```python
from build123d import *

# Parameters (mm, degrees)
F1_DEPTH = 63.5
F2_DEPTH = 25.4
F3_DEPTH = 7.9375


with BuildPart() as f1:
    # F0 (on Front) → F1 (new body, symmetric)
    with BuildSketch(Plane.XZ):
        Polygon((-41.275, 9.525), (-41.275, -9.525), (41.275, -9.525), (41.275, 9.525), (22.225, 9.525), align=None)
    extrude(amount=F1_DEPTH, both=True)

    # F0 (on Front) → F2 (join, symmetric)
    with BuildSketch(Plane.XZ):
        with BuildLine():
            Line((22.225, 9.525), (41.275, 9.525))
            Line((41.275, 9.525), (41.275, 27.144268))
            ThreePointArc((41.275, 27.144268), (46.70633, 39.100244), (59.283867, 42.8752))
            Line((59.283867, 42.8752), (60.325, 42.8752))
            Line((60.325, 42.8752), (60.325, 61.9252))
            Line((60.325, 61.9252), (60.318968, 61.9252))
            add(Edge.make_bspline(
                [(60.318968, 61.9252), (58.637809, 61.975807), (56.975817, 62.007969), (55.33311, 62.021976)],
                knots=[0, 0, 0, 0, 3.185994, 3.185994, 3.185994, 3.185994], degree=3))
            ThreePointArc((55.33311, 62.021976), (31.820072, 51.189025), (22.225, 27.144268))
            Line((22.225, 27.144268), (22.225, 9.525))
        make_face()
        Polygon((60.325, 66.675), (60.325, 61.9252), (60.325, 42.8752), (85.883424, 42.8752), (85.578844, 66.675), align=None)
    extrude(amount=F2_DEPTH, both=True)

    # F0 (on Front) → F3 (join, symmetric)
    with BuildSketch(Plane.XZ):
        with BuildLine():
            add(Edge.make_bspline(
                [(55.33311, 62.021976), (-1.963501, 62.510512), (-35.799797, 40.911554), (-41.275, 9.525)],
                knots=[3.185994, 3.185994, 3.185994, 3.185994, 114.311484, 114.311484, 114.311484, 114.311484], degree=3))
            Line((-41.275, 9.525), (22.225, 9.525))
            Line((22.225, 9.525), (22.225, 27.144268))
            ThreePointArc((22.225, 27.144268), (31.820072, 51.189025), (55.33311, 62.021976))
        make_face()
    extrude(amount=F3_DEPTH, both=True)


solid = f1.part
```
Model file for the job. Use its own axes, mm. A direction names the side the tool comes from. Coordinates: 2 decimals unless noted, no trailing zeros. Loops run counter-clockwise (first coordinate to the right, second up) from the corner with the lowest first, then second, coordinate; pieces in that order, holes last. Notation, with made-up numbers: (-23, -23) - (-19, -23) arc R29 cw to (-19, 15) - close; hole circle Ø5 at (-19.5, 49). An arc over 180 degrees is marked (long way). Answer as a JSON object with one key per item and string values. Group by question number.
(1) Tool access for faces 1 (the face through (22.225, -17, 18)), 2 (the face through (22.225, 17, 18)), 3 (the face through (54, -25.4, 45)), 4 (the face through (54, 25.4, 45)): list every direction of +Z, -Z, +X, -X, +Y, -Y with a clear straight run to the whole face (end or side of a thin tool).
(2) Probe line 1 along Z through (x, y) = (-34, 40) (3 decimals); line 2 along Z through (x, y) = (78.5, 24.5) (3 decimals); line 3 along Y through (x, z) = (-13, 35.5). List the from-to ranges inside material, lowest first.
(3) Flat gauge pins, fed straight in: pin 1 (1.4 mm diameter, centred on y = -10, z = 65, fed in from -X) (3 decimals); pin 2 (2 mm diameter, centred on y = -1.5, z = 52, fed in from -X); pin 3 (14 mm diameter, centred on y = 20.5, z = 20.5, fed in from -X) (3 decimals). Where does each tip first touch, or does it go through?
(4) Cut at B-B (y = 53.5). Give the cut face in (x, z) (3 decimals), then the cut area to 3 significant figures.
(5) Cut at A-A (z = -1). Give the cut face in (x, y) (3 decimals), then the cut area to 3 significant figures.
Geometry says:
{
 "1": {"face 1": "+Z, -X, -Y", "face 2": "+Z, -X, +Y", "face 3": "+Z, +X, -X, -Y", "face 4": "+Z, +X, -X, +Y"},
 "2": {"line 1": "z = -9.525 to 9.525", "line 2": "z = 42.875 to 66.675", "line 3": "y = -7.94 to 7.94"},
 "3": {"pin 1": "stops at x = 60.325", "pin 2": "stops at x = -6.01", "pin 3": "stops at x = 22.225"},
 "4": {"outline": "(-41.275, -9.525) - (41.275, -9.525) - (41.275, 9.525) - (-41.275, 9.525) - close", "area": "1,570 mm^2"},
 "5": {"outline": "(-41.275, -63.5) - (41.275, -63.5) - (41.275, 63.5) - (-41.275, 63.5) - close", "area": "10,500 mm^2"}
}
